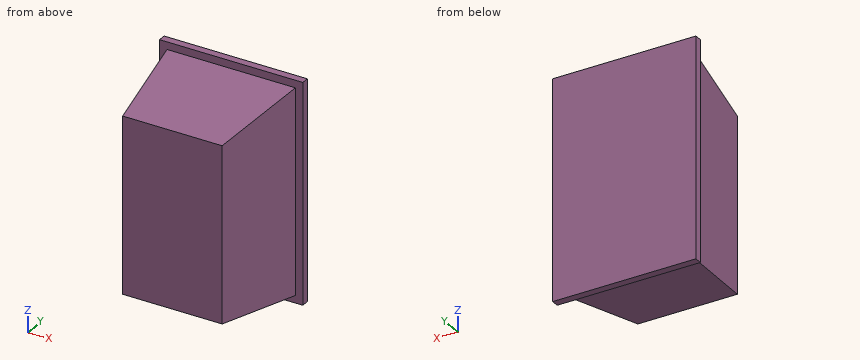
from build123d import *

# Parameters (mm, degrees)
F1_DEPTH = 746.125
F3_DEPTH = 488.951


with BuildPart() as f1:
    # F0 (on Top) → F1 (new body)
    with BuildSketch(Plane.XY):
        Polygon((366.779292, 60.914483), (-71.370708, 60.914483), (-22.158208, -269.285517), (317.566792, -269.285517), align=None)
        Polygon((-96.770708, 60.914483), (-71.370708, 60.914483), (366.779292, 60.914483), (392.179292, 60.914483), (392.179292, 86.314483), (-96.770708, 86.314483), align=None)
    extrude(amount=F1_DEPTH)

    # F2 (on face) → F3 (cut, through all)
    with BuildSketch(Plane.YZ.offset(392.179292)):
        Polygon((60.914483, 720.725), (60.914483, 746.125), (-269.285517, 746.125), (-269.285517, 671.4998), align=None)
        Polygon((-269.285517, 74.6252), (-269.285517, 0), (60.914483, 0), (60.914483, 25.4), align=None)
    extrude(amount=-F3_DEPTH, mode=Mode.SUBTRACT)


solid = f1.part
For this review, take the finished solid that the model builds, in its own axes (mm). Round coordinates to 2 decimals unless told otherwise and drop trailing zeros. Write each loop counter-clockwise with the first axis right and the second up, starting at its lowest first coordinate (ties: lowest second). Pieces come first, ordered by that corner, then holes. Notation, with made-up numbers: (-16, 54.25) - (-11, 54.25) arc R16 cw to (-11, 63.25) - close; hole circle Ø2 at (56, 25.5). An arc over 180 degrees is marked (long way). Write item = value, one per line. Start each with the question number.
1. Consider section D-D on y = -182. State the section outline as (x, z) points, plus the area to 3 significant figures.
2. Consider section B-B on x = 23.5. State the section outline as (y, z) points (3 decimals), plus the area to 3 significant figures.
3. Consider section A-A on z = 171. State the section outline as (x, y) points.
4. Wall thickness on L1, parallel to X at y = 7.5, z = 255; L2, parallel to Z at x = 32, y = -99.5; L3, parallel to Z at x = 115, y = -190: over which ranges is each line inside the solid? List them lowest first.
5. For pin 1 Ø2 at (x, y) = (98.5, -122) entering from -Z; pin 2 Ø3 at (y, z) = (-211.5, 412) entering from +X; pin 3 Ø6 at (y, z) = (-69.5, 313) entering from -X, all flat-tipped, find the tip position at first contact; note any pin that passes through.
6. Consider section C-C on y = -145. State the section outline as (x, z) points.
Evaluation:
q1.outline = (-35.17, 61.61) - (330.58, 61.61) - (330.58, 684.51) - (-35.17, 684.51) - close
q1.area = 228,000 mm2
q2.outline = (-269.286, 74.625) - (60.914, 25.4) - (60.914, 0) - (86.314, 0) - (86.314, 746.125) - (60.914, 746.125) - (60.914, 720.725) - (-269.286, 671.5) - close
q2.area = 232,000 mm2
q3.outline = (-96.77, 60.91) - (-71.37, 60.91) - (-22.16, -269.29) - (317.57, -269.29) - (366.78, 60.91) - (392.18, 60.91) - (392.18, 86.31) - (-96.77, 86.31) - close
q4.L1 = -63.41 to 358.82
q4.L2 = 49.31 to 696.81
q4.L3 = 62.81 to 683.32
q5.pin_1 = 52.52
q5.pin_2 = 326.4
q5.pin_3 = -52.38
q6.outline = (-40.68, 56.1) - (336.09, 56.1) - (336.09, 690.03) - (-40.68, 690.03) - close
